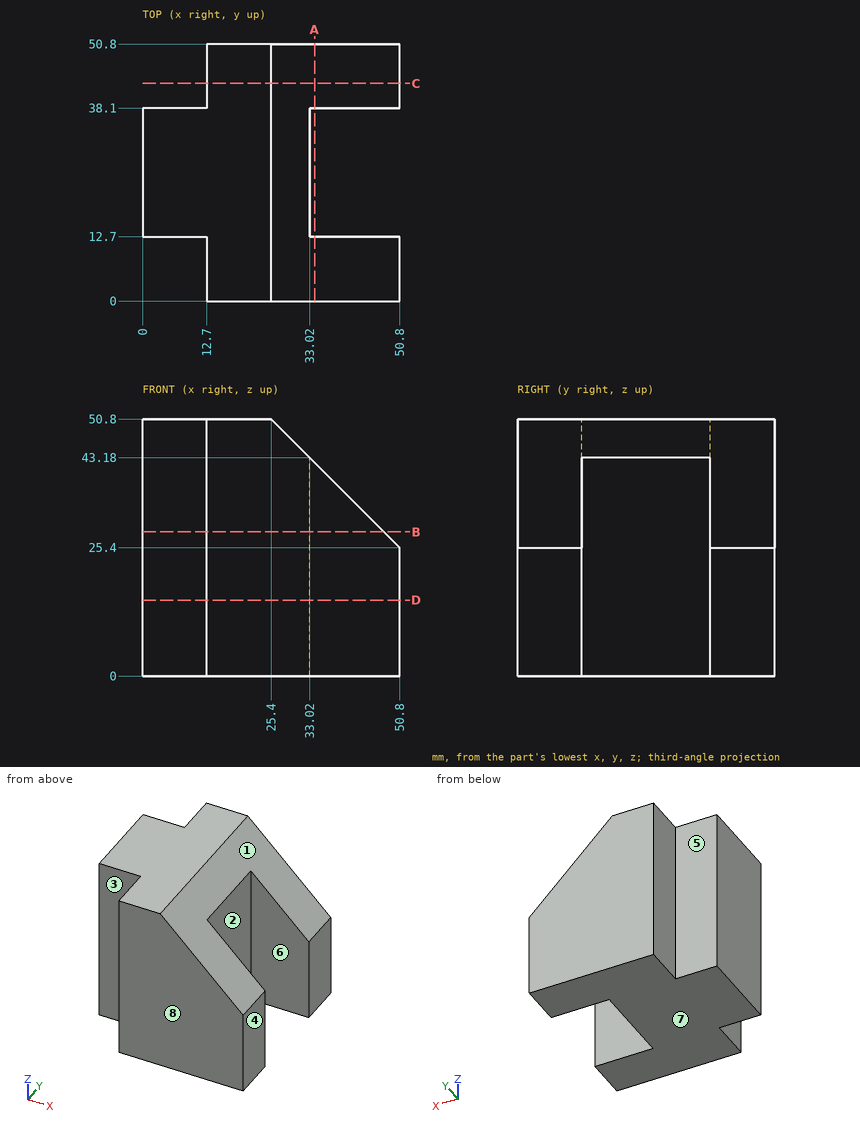
Verification items for this drawing (mm, ordinates from the low corner). A direction names the side the tool comes from. Round coordinates to 2 decimals unless told otherwise and drop trailing zeros. Loops run counter-clockwise (first coordinate to the right, second up) from the corner with the lowest first, then second, coordinate; pieces in that order, holes last. Notation, with made-up numbers: (-13, -36.75) -> (8, -36.75) arc R12 ccw to (8, -17.75) -> close; hole circle Ø3 at (58.25, -24). An arc over 180 degrees is marked (long way). Answer in a Markdown table with one row per item.
Q1. Sectioned sample at B-B on z = 28.5. Enter the section's corners in (x, y).
Data:
| item | result |
|---|---|
| outline | (0, 12.7) -> (12.7, 12.7) -> (12.7, 0) -> (47.7, 0) -> (47.7, 12.7) -> (33.02, 12.7) -> (33.02, 38.1) -> (47.7, 38.1) -> (47.7, 50.8) -> (12.7, 50.8) -> (12.7, 38.1) -> (0, 38.1) -> close |
Q2. Thickness scan on L1, parallel to Y at x = 42, z = 20; L2, parallel to X at y = 38, z = 7; L3, parallel to Y at x = 10.5, z = 21.5. Record the ranges inside material, lowest first.
Data:
| item | result |
|---|---|
| L1 | y = 0 to 12.7, 38.1 to 50.8 |
| L2 | x = 0 to 33.02 |
| L3 | y = 12.7 to 38.1 |
Q3. Sectioned sample at D-D on z = 15. Enter the section's corners in (x, y), then the cut area to 3 significant figures.
Data:
| item | result |
|---|---|
| outline | (0, 12.7) -> (12.7, 12.7) -> (12.7, 0) -> (50.8, 0) -> (50.8, 12.7) -> (33.02, 12.7) -> (33.02, 38.1) -> (50.8, 38.1) -> (50.8, 50.8) -> (12.7, 50.8) -> (12.7, 38.1) -> (0, 38.1) -> close |
| area | 1,810 mm^2 |
Q4. Go/stop test with flat-tipped pins: P1, Ø12.5, axis at y = 22.5, z = 16.5, coming from the +X side; P2, Ø4, axis at x = 4, z = 19.5, coming from the +Y side; P3, Ø10, axis at x = 7.5, z = 23, coming from the -Y side. Record where each tip stops, or that it passes through.
Data:
| item | result |
|---|---|
| P1 | stops at x = 33.02 |
| P2 | stops at y = 38.1 |
| P3 | stops at y = 12.7 |
Q5. Sectioned sample at A-A on x = 34. Enter the section's corners in (y, z), then the cut area to 3 significant figures.
Data:
| item | result |
|---|---|
| outline | (0, 0) -> (12.7, 0) -> (12.7, 42.2) -> (0, 42.2) -> close; (38.1, 0) -> (50.8, 0) -> (50.8, 42.2) -> (38.1, 42.2) -> close |
| area | 1,070 mm^2 |
Q6. Sectioned sample at C-C on y = 43. Enter the section's corners in (x, z), then the cut area to 3 significant figures.
Data:
| item | result |
|---|---|
| outline | (12.7, 0) -> (50.8, 0) -> (50.8, 25.4) -> (25.4, 50.8) -> (12.7, 50.8) -> close |
| area | 1,610 mm^2 |
Q7. Release check for a two-part mould opening along Y. For the marked faces 6, 7 and 8 record: released by +Y, released by -Y, zero draft, split by the parting line, or undercut.
Data:
| item | result |
|---|---|
| face 6 | undercut |
| face 7 | zero draft |
| face 8 | released by -Y |
Q8. Set-up check for the marked faces 1, 2, 3, 4 and 5: record each of +Z, -Z, +X, -X, +Y, -Y from which the full face is reachable in a straight line by a thin tool's end or side.
Data:
| item | result |
|---|---|
| face 1 | +Z, +X, +Y, -Y |
| face 2 | +Z, -Z, +X |
| face 3 | +Z, -Z, -X, -Y |
| face 4 | +Z, -Z, +X, +Y, -Y |
| face 5 | +Z, -Z, -X, +Y |
